from build123d import *

# Parameters (mm, degrees)
SKETCH1_W           = 52
SKETCH1_H           = 37
SKETCH1_W_2         = 50
SKETCH1_H_2         = 35
BOSS_EXTRUDE1_DEPTH = 30
SKETCH2_W           = 52
SKETCH2_H           = 37
BOSS_EXTRUDE2_DEPTH = 2
CUT_EXTRUDE1_DEPTH  = 2
SKETCH4_W           = 50
SKETCH4_H           = 2
BOSS_EXTRUDE3_DEPTH = 2
CUT_EXTRUDE2_REACH  = 54
SKETCH7_W           = 50
SKETCH7_H           = 1
BOSS_EXTRUDE4_DEPTH = 19


with BuildPart() as part:
    # Sketch1 → Boss-Extrude1 (new body)
    with BuildSketch(Plane(origin=(0, 0, 0), x_dir=(1, 0, 0), z_dir=(0, 1, 0))):
        with Locations((26, 18.5)):
            Rectangle(SKETCH1_W, SKETCH1_H)
        with Locations((26, 18.5)):
            Rectangle(SKETCH1_W_2, SKETCH1_H_2, mode=Mode.SUBTRACT)
    extrude(amount=BOSS_EXTRUDE1_DEPTH)

    # Sketch2 → Boss-Extrude2 (add)
    with BuildSketch(Plane(origin=(0, 0, 0), x_dir=(1, 0, 0), z_dir=(0, 1, 0))):
        with Locations((26, 18.5)):
            Rectangle(SKETCH2_W, SKETCH2_H)
    extrude(amount=BOSS_EXTRUDE2_DEPTH)

    # Sketch3 → Cut-Extrude1 (cut)
    with BuildSketch(Plane.XY):
        with BuildLine():
            Line((4.85, 12), (4.85, 30))
            Line((4.85, 30), (20.85, 30))
            Line((20.85, 30), (20.85, 12))
            ThreePointArc((20.85, 12), (12.85, 4), (4.85, 12))
        make_face()
        with BuildLine():
            Line((31.15, 12), (31.15, 30))
            Line((31.15, 30), (47.15, 30))
            Line((47.15, 30), (47.15, 12))
            ThreePointArc((47.15, 12), (39.15, 4), (31.15, 12))
        make_face()
    extrude(amount=-CUT_EXTRUDE1_DEPTH, mode=Mode.SUBTRACT)

    # Sketch4 → Boss-Extrude3 (add)
    with BuildSketch(Plane(origin=(0, 2, 0), x_dir=(1, 0, 0), z_dir=(0, 1, 0))):
        with Locations((26, 6.5)):
            Rectangle(SKETCH4_W, SKETCH4_H)
        with Locations((26, 14.5)):
            Rectangle(SKETCH4_W, SKETCH4_H)
        with Locations((26, 18.25)):
            Rectangle(SKETCH4_W, SKETCH4_H)
    extrude(amount=BOSS_EXTRUDE3_DEPTH)

    # Sketch5 → Cut-Extrude2 (cut, up to next)
    with BuildSketch(Plane(origin=(52, 0, 0), x_dir=(0, 0, -1), z_dir=(1, 0, 0)), mode=Mode.PRIVATE) as cut_extrude2_sk1:
        with BuildLine():
            Line((30.5, 30), (22.5, 30))
            Line((22.5, 30), (22.5, 12))
            ThreePointArc((22.5, 12), (23.085786438, 10.585786438), (24.5, 10))
            Line((24.5, 10), (28.5, 10))
            ThreePointArc((28.5, 10), (29.914213562, 10.585786438), (30.5, 12))
            Line((30.5, 12), (30.5, 30))
        make_face()
    cut_extrude2_tool1 = extrude(cut_extrude2_sk1.sketch, amount=-CUT_EXTRUDE2_REACH, mode=Mode.PRIVATE) & part.part
    add(cut_extrude2_tool1.solids().sort_by_distance((52, 20.103619, -26.5))[0], mode=Mode.SUBTRACT)

    # Sketch7 → Boss-Extrude4 (add)
    with BuildSketch(Plane(origin=(0, 2, 0), x_dir=(1, 0, 0), z_dir=(0, 1, 0))):
        with Locations((26, 8)):
            Rectangle(SKETCH7_W, SKETCH7_H)
    extrude(amount=BOSS_EXTRUDE4_DEPTH)


solid = part.part
Verification items for the finished model (mm, model axes). A direction names the side the tool comes from. Give positions to 0.01 mm unless a question says otherwise; leave off trailing zeros. Order: outer loops, then holes, each group sorted by start corner. A loop starts at its lowest first (then second) coordinate and runs counter-clockwise, first axis right, second up. Notation, with made-up numbers: M -16,34 L 41,34 A22 ccw 41,66 Z; hole C 50,-6.5 d7. An arc over 180 degrees is marked long. Use one line per item in the form item = value. Start each with the question number.
Q1. Scan lines: line 1 along Z through (x, y) = (23, 17.5); line 2 along Z through (x, y) = (24, 3); line 3 along X through (y, z) = (28.25, -17). Record each from-to range of solid material in increasing order. Write a range as [from, to].
Q2. Access from +Z, -Z, +X, -X, +Y, -Y to the whole of each face (thin tool, end or side, straight path). Record for faces 4 (the flat face through (0, 15, -18)), 5 (the flat face through (26, 3, -15.5)), 6 (the cylindrical face through (13, 4, -0.5)).
Q3. Mould release check, pull along X, two halves, no side actions. Record for faces 1 (the flat face through (26, 3, -13.5)), 2 (the flat face through (52, 15, -18)), 3 (the cylindrical face through (51.51, 10.6, -23.07)): +X half, -X half, draft (parallel to the pull), parting line (faces both ways), or undercut.
Q4. Section check B-B (y = 25.25). Enter the section's corners in (x, z).
Q5. Section check D-D (y = 18.5). Enter the section's corners in (x, z), then the cut area to 3 significant figures.
Q6. Go/stop test with flat-tipped pins: pin 1 Ø10 at (x, z) = (12, -5) entering from +Y; pin 2 Ø2 at (x, z) = (20, -18) entering from +Y; pin 3 Ø1.5 at (x, y) = (8, 14) entering from +Z. Record where each tip stops, or that it passes through.
Q7. Section check C-C (z = -34). Enter the section's corners in (x, y), then the cut area to 3 significant figures.
Q8. Section check A-A (y = 9.25). Enter the section's corners in (x, z), then the cut area to 3 significant figures.
Evaluation:
q1.line_1 = [-37, -36], [-8.5, -7.5], [-1, 0]
q1.line_2 = [-37, -36], [-19.25, -17.25], [-15.5, -13.5], [-8.5, -5.5], [-1, 0]
q1.line_3 = [0, 1], [51, 52]
q2.face_4 = +Z, -Z, -X, +Y, -Y
q2.face_5 = +Y
q2.face_6 = +Z, +Y
q3.face_1 = undercut
q3.face_2 = +X half
q3.face_3 = draft
q4.outline = M 0,-37 L 52,-37 L 52,-30.5 L 51,-30.5 L 51,-36 L 1,-36 L 1,-1 L 4.85,-1 L 4.85,0 L 0,0 Z; M 20.85,-1 L 31.15,-1 L 31.15,0 L 20.85,0 Z; M 47.15,-1 L 51,-1 L 51,-22.5 L 52,-22.5 L 52,0 L 47.15,0 Z
q5.outline = M 0,-37 L 52,-37 L 52,-30.5 L 51,-30.5 L 51,-36 L 1,-36 L 1,-8.5 L 51,-8.5 L 51,-22.5 L 52,-22.5 L 52,0 L 47.15,0 L 47.15,-1 L 51,-1 L 51,-7.5 L 1,-7.5 L 1,-1 L 4.85,-1 L 4.85,0 L 0,0 Z; M 20.85,-1 L 31.15,-1 L 31.15,0 L 20.85,0 Z
q5.area = 184 mm2
q6.pin_1 = 21
q6.pin_2 = 4
q6.pin_3 = -7.5
q7.outline = M 0,0 L 52,0 L 52,30 L 51,30 L 51,2 L 1,2 L 1,30 L 0,30 Z
q7.area = 160 mm2
q8.outline = M 0,-37 L 52,-37 L 52,0 L 46.66,0 L 46.66,-1 L 51,-1 L 51,-7.5 L 1,-7.5 L 1,-1 L 5.34,-1 L 5.34,0 L 0,0 Z; M 20.36,-1 L 31.64,-1 L 31.64,0 L 20.36,0 Z; hole M 1,-36 L 51,-36 L 51,-8.5 L 1,-8.5 Z
q8.area = 194 mm2
